from build123d import *

# Parameters (mm, degrees)
PAD009_DEPTH         = 5.5
SKETCH015_R          = 1.5
PAD010_DEPTH         = 7.5
SKETCH016_W          = 5.8
SKETCH016_H          = 5.8
POCKET005_DEPTH      = 1.501
POCKET005_DEPTH_BACK = 3.001
SKETCH019_W          = 6.5
SKETCH019_H          = 6.5
POCKET006_DEPTH      = 1.501
SKETCH017_R          = 1.1
PAD011_DEPTH         = 2


with BuildPart() as part:
    # Sketch014 → Pad009 (new body, symmetric)
    with BuildSketch(Plane.XZ):
        with BuildLine():
            ThreePointArc((14.36977, 3), (13.850991, 0.778814), (13.95, -1.5))
            Line((13.95, -1.5), (30.45, -1.5))
            ThreePointArc((30.45, -1.5), (30.549009, 0.778814), (30.03023, 3))
            Line((30.03023, 3), (25.7, 2))
            Line((18.7, 2), (25.7, 2))
            Line((14.36977, 3), (18.7, 2))
        make_face()
    extrude(amount=PAD009_DEPTH, both=True)

    # Sketch015 → Pad010 (join, symmetric)
    with BuildSketch(Plane.XZ):
        with Locations((22.2, 0)):
            Circle(SKETCH015_R)
    extrude(amount=PAD010_DEPTH, both=True)

    # Sketch016 → Pocket005 (cut, two sides)
    with BuildSketch(Plane.XY) as pocket005_sk:
        with Locations((22.2, 0)):
            Rectangle(SKETCH016_W, SKETCH016_H)
    extrude(amount=-POCKET005_DEPTH, mode=Mode.SUBTRACT)
    extrude(pocket005_sk.sketch, amount=POCKET005_DEPTH_BACK, mode=Mode.SUBTRACT)

    # Sketch019 → Pocket006 (cut, through all)
    with BuildSketch(Plane.XY):
        with Locations((22.2, 0)):
            Rectangle(SKETCH019_W, SKETCH019_H)
    extrude(amount=-POCKET006_DEPTH, mode=Mode.SUBTRACT)

    # Sketch017 → Pad011 (join)
    with BuildSketch(Plane.XY):
        with Locations((15.2, 0)):
            Circle(SKETCH017_R)
        with Locations((29.2, 0)):
            Circle(SKETCH017_R)
    extrude(amount=-PAD011_DEPTH)


with BuildPart() as part_1:
    # Body005 placement: moved
    add(part.part.moved(Location((0, 32.5, 8.5))))


solid = part_1.part
For this review, take the finished solid that the model builds, in its own axes (mm). A direction names the side the tool comes from. Give positions to 0.01 mm unless a question says otherwise; leave off trailing zeros. Order: outer loops, then holes, each group sorted by start corner. A loop starts at its lowest first (then second) coordinate and runs counter-clockwise, first axis right, second up. Notation, with made-up numbers: (88, 44) - (97, 44) arc R18 cw to (97, 64) - close; hole circle Ø10 at (45, 21.25). An arc over 180 degrees is marked (long way). Answer as a JSON object with one key per item and string values. Group by question number.
Item 1: Wall thickness on line 1 along Y through (x, z) = (22.5, 8.25); line 2 along X through (y, z) = (26.5, 8.5); line 3 along Y through (x, z) = (27.75, 9.2): over which ranges is each line inside the solid? List them lowest first.
Item 2: Draft analysis for pull direction Y (two halves, no side actions). For faces 5 (the flat face through (22, 36, 7)), 6 (the flat face through (22.1, 38, 10.3)), 7 (the flat face through (22, 29.25, 8)), state which applies: pulls with the +Y half, pulls with the -Y half, needs draft (parallel to the pull), parting line crosses it, or undercut.
Item 3: Take a section at B-B on x = 21. Give the boundary of the cut face in (y, z).
Item 4: Take a section at D-D on z = 10.75. Give the boundary of the cut face in (x, y).
Item 5: Machinability: for faces 1 (the cylindrical face through (15.79, 33.43, 6.75)), 2 (the flat face through (25.1, 32, 9)), 3 (the cylindrical face through (21.875, 38.986, 7.036)), 4 (the cylindrical face through (21.875, 25.986, 7.036)), which of the approach directions +Z, -Z, +X, -X, +Y, -Y give a long, thin tool a straight path to every point of the face, cutting with its end or side? Answer none if there is none.
Item 6: Clearance check with flat-ended pins moving along their axes: pin 1 Ø3.5 at (x, y) = (19.5, 33) entering from -Z; pin 2 Ø3 at (x, y) = (22.5, 32) entering from -Z; pin 3 Ø1.6 at (y, z) = (33.5, 10) entering from +X; pin 4 Ø0.6 at (y, z) = (33.5, 9.5) entering from -X. State where each tip first meets the part, or that it passes through.
Item 7: Take a section at A-A on y = 32.5. Give the boundary of the cut face in (x, z).
Item 8: Take a section at C-C on z = 8.1. Give the boundary of the cut face in (x, y), and give its area (3 significant figures).
Reported:
{
 "1": {"line 1": "25 to 29.25, 35.75 to 40", "line 2": "20.7 to 23.7", "line 3": "27 to 38"},
 "2": {"face 5": "needs draft", "face 6": "pulls with the +Y half", "face 7": "undercut"},
 "3": {"outline": "(25, 7.6) - (27, 7.6) - (27, 7) - (29.25, 7) - (29.25, 8.5) - (29.6, 8.5) - (29.6, 10.5) - (27, 10.5) - (27, 9.4) - (25, 9.4) - close; (35.4, 8.5) - (35.75, 8.5) - (35.75, 7) - (38, 7) - (38, 7.6) - (40, 7.6) - (40, 9.4) - (38, 9.4) - (38, 10.5) - (35.4, 10.5) - close"},
 "4": {"outline": "(14.12, 27) - (17.62, 27) - (17.62, 38) - (14.12, 38) - close; (26.78, 27) - (30.28, 27) - (30.28, 38) - (26.78, 38) - close"},
 "5": {"face 1": "-Z", "face 2": "+Z, -Z", "face 3": "+Y", "face 4": "-Y"},
 "6": {"pin 1": "z = 7", "pin 2": "through", "pin 3": "x = 30.56", "pin 4": "x = 13.84"},
 "7": {"outline": "(13.95, 7) - (14.1, 7) - (14.1, 6.5) - (16.3, 6.5) - (16.3, 7) - (18.95, 7) - (18.95, 8.5) - (19.3, 8.5) - (19.3, 10.5) - (18.7, 10.5) - (14.37, 11.5) arc R8.39 ccw to start; (25.1, 8.5) - (25.45, 8.5) - (25.45, 7) - (28.1, 7) - (28.1, 6.5) - (30.3, 6.5) - (30.3, 7) - (30.45, 7) arc R8.39 ccw to (30.03, 11.5) - (25.7, 10.5) - (25.1, 10.5) - close"},
 "8": {"outline": "(13.82, 27) - (20.75, 27) - (20.75, 25) - (23.65, 25) - (23.65, 27) - (30.58, 27) - (30.58, 38) - (23.65, 38) - (23.65, 40) - (20.75, 40) - (20.75, 38) - (13.82, 38) - close; hole (18.95, 29.25) - (25.45, 29.25) - (25.45, 35.75) - (18.95, 35.75) - close", "area": "154 mm^2"}
}
